Part print with two shaded views. Sizes in mm from the minimum x, y, z corner. Round coordinates to 2 decimals unless told otherwise and drop trailing zeros. Loops run counter-clockwise (first coordinate to the right, second up) from the corner with the lowest first, then second, coordinate; pieces in that order, holes last.
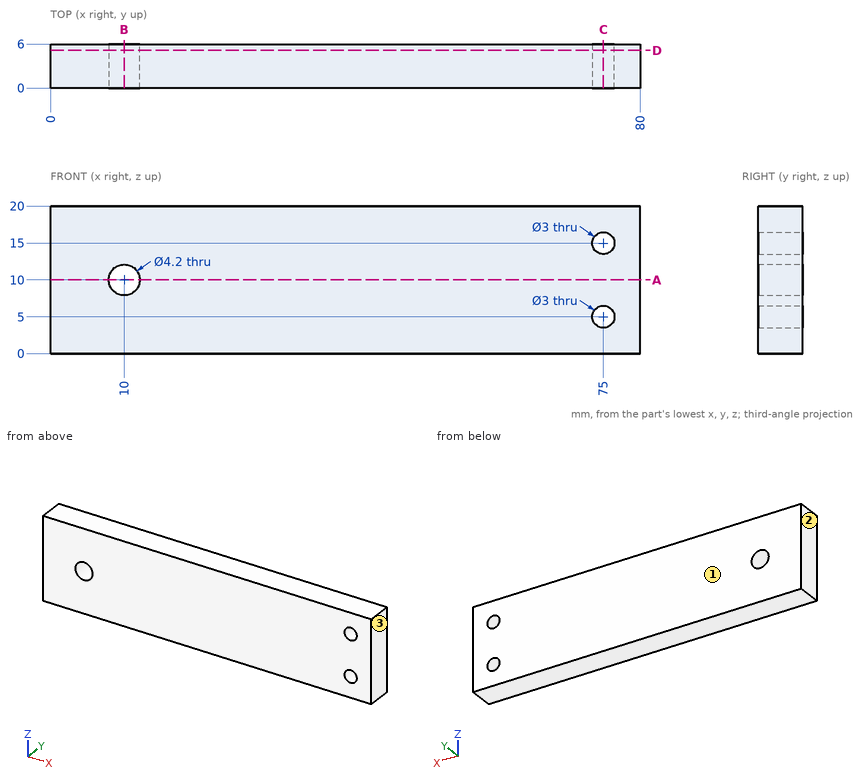
Item 1: Cut at B-B (x = 10). List the corners of the cut face in (y, z), plus the area to 3 significant figures.
Verdict:
outline: (0, 0) - (6, 0) - (6, 7.9) - (0, 7.9) - close; (0, 12.1) - (6, 12.1) - (6, 20) - (0, 20) - close
area: 94.8 mm2
Item 2: Mould opens along X. For the marked faces 1, 2 and 3 say: released by +X, released by -X, zero draft, split by the parting line, or undercut.
Verdict:
face 1: zero draft
face 2: released by -X
face 3: released by +X
Item 3: Wall check: L1, parallel to Z at x = 75, y = 3.8; L2, parallel to Z at x = 10, y = 2.6; L3, parallel to X at y = 4.4, z = 10.25. Give the ranges that are in metal, low to high.
Verdict:
L1: z = 0 to 3.5, 6.5 to 13.5, 16.5 to 20
L2: z = 0 to 7.9, 12.1 to 20
L3: x = 0 to 7.91, 12.09 to 80
Item 4: Cut at C-C (x = 75). List the corners of the cut face in (y, z).
Verdict:
outline: (0, 0) - (6, 0) - (6, 3.5) - (0, 3.5) - close; (0, 6.5) - (6, 6.5) - (6, 13.5) - (0, 13.5) - close; (0, 16.5) - (6, 16.5) - (6, 20) - (0, 20) - close
Item 5: Cut at D-D (y = 5.15). List the corners of the cut face in (x, z).
Verdict:
outline: (0, 0) - (80, 0) - (80, 20) - (0, 20) - close; hole circle Ø4.2 at (10, 10); hole circle Ø3 at (75, 5); hole circle Ø3 at (75, 15)
Item 6: Cut at A-A (z = 10). List the corners of the cut face in (x, y), plus the area to 3 significant figures.
Verdict:
outline: (0, 0) - (7.9, 0) - (7.9, 6) - (0, 6) - close; (12.1, 0) - (80, 0) - (80, 6) - (12.1, 6) - close
area: 455 mm2
Item 7: Flat gauge pin, fed straight in: P1, Ø2, axis at x = 49.5, y = 3, coming from the -Z side. Where does the tip first touch, or does it go through?
Verdict:
P1: stops at z = 0
